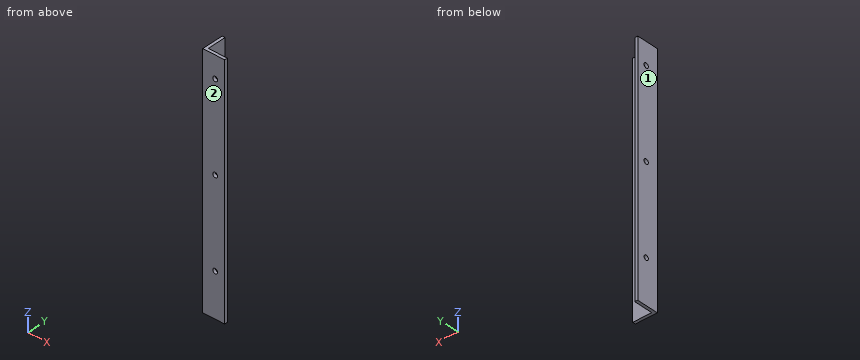
from build123d import *

# Parameters (mm, degrees)
EXTRUDE_1_DEPTH          = 150
EXTRUDE_2_DEPTH          = 15
M4X0_7_1_D               = 3.3
M4X0_7_1_DEPTH           = 11.5
M4X0_7_1_TIP             = 0.991420021
M4X0_7_1_ON_FACE_2_D     = 3.3
M4X0_7_1_ON_FACE_2_DEPTH = 11.5
M4X0_7_1_ON_FACE_2_TIP   = 0.991420021


with BuildPart() as part:
    # ｽｹｯﾁ1 → ﾎﾞｽ - 押し出し1 (new body)
    with BuildSketch(Plane.XY):
        Polygon((0, 0), (0, 15), (2, 15), (2, 2), (15, 2), (15, 0), align=None)
    extrude(amount=EXTRUDE_1_DEPTH)

    # ｽｹｯﾁ7 → ﾎﾞｽ - 押し出し2 (add)
    with BuildSketch(Plane(origin=(0, 0, 0), x_dir=(-1, 0, 0), z_dir=(0, 0, -1))):
        Polygon((-15, 2), (-2, 2), (-2, 15), (0, 15), (0, 0), (-15, 0), align=None)
    extrude(amount=EXTRUDE_2_DEPTH)

    # M4x0.7 ねじ穴1
    with Locations(Plane(origin=(8.5, 2, 15), x_dir=(0, 0, 1), z_dir=(0, 1, 0))):
        with Locations((0, 0), (60, 0), (120, 0)):
            Hole(M4X0_7_1_D / 2, depth=M4X0_7_1_DEPTH)
            with Locations((0, 0, -(M4X0_7_1_DEPTH + M4X0_7_1_TIP / 2))):  # 118° drill point
                Cone(0, M4X0_7_1_D / 2, M4X0_7_1_TIP, mode=Mode.SUBTRACT)

    # M4x0.7 ねじ穴1 on face 2
    with Locations(Plane(origin=(2, 8.5, 135), x_dir=(0, 0, 1), z_dir=(1, 0, 0))):
        with Locations((0, 0), (-60, 0), (-120, 0)):
            Hole(M4X0_7_1_ON_FACE_2_D / 2, depth=M4X0_7_1_ON_FACE_2_DEPTH)
            with Locations((0, 0, -(M4X0_7_1_ON_FACE_2_DEPTH + M4X0_7_1_ON_FACE_2_TIP / 2))):  # 118° drill point
                Cone(0, M4X0_7_1_ON_FACE_2_D / 2, M4X0_7_1_ON_FACE_2_TIP, mode=Mode.SUBTRACT)


solid = part.part
Geometry: final body of the model. Coordinates: model frame, mm. Face numbers are marked on the shaded views. Coordinates: 2 decimals unless noted, no trailing zeros. Order: outer loops, then holes, each group sorted by start corner. A loop starts at its lowest first (then second) coordinate and runs counter-clockwise, first axis right, second up.
(1) Section query D-D (z = -0.5). Return the cut outline in (x, y).
(2) Section query A-A (z = 75). Return the cut outline in (x, y), plus the area to 3 significant figures.
(3) Section query B-B (x = 8.5). Return the cut outline in (y, z).
(4) Material intervals for probe 1 along Z at (x, y) = (1.05, 8.5); probe 2 along X at (y, z) = (1.35, 15), sorted ascending.
(5) First-contact query: pin 1 (6.5 mm diameter, centred on y = 6, z = 106, fed in from +X); pin 2 (2.5 mm diameter, centred on x = 8.5, z = 75, fed in from +Y); pin 3 (4 mm diameter, centred on x = 9.5, z = 42.5, fed in from +Y). Flat tips, straight axial feed; report the tip coordinate or a pass-through.
(6) Draft query along X for the marked faces 1 and 2. Return one class per face: pulls with the +X half, pulls with the -X half, needs draft (parallel to the pull), parting line crosses it, or undercut.
Solution:
1. outline: (0, 0) - (15, 0) - (15, 2) - (2, 2) - (2, 15) - (0, 15) - close
2. outline: (0, 0) - (6.85, 0) - (6.85, 2) - (2, 2) - (2, 6.85) - (0, 6.85) - close; (0, 10.15) - (2, 10.15) - (2, 15) - (0, 15) - close; (10.15, 0) - (15, 0) - (15, 2) - (10.15, 2) - close
2. area: 42.8 mm2
3. outline: (0, -15) - (2, -15) - (2, 13.35) - (0, 13.35) - close; (0, 16.65) - (2, 16.65) - (2, 73.35) - (0, 73.35) - close; (0, 76.65) - (2, 76.65) - (2, 133.35) - (0, 133.35) - close; (0, 136.65) - (2, 136.65) - (2, 150) - (0, 150) - close
4. probe 1: z = -15 to 13.35, 16.65 to 73.35, 76.65 to 133.35, 136.65 to 150
4. probe 2: x = 0 to 6.85, 10.15 to 15
5. pin 1: stops at x = 2
5. pin 2: passes through
5. pin 3: stops at y = 2
6. face 1: pulls with the -X half
6. face 2: needs draft
